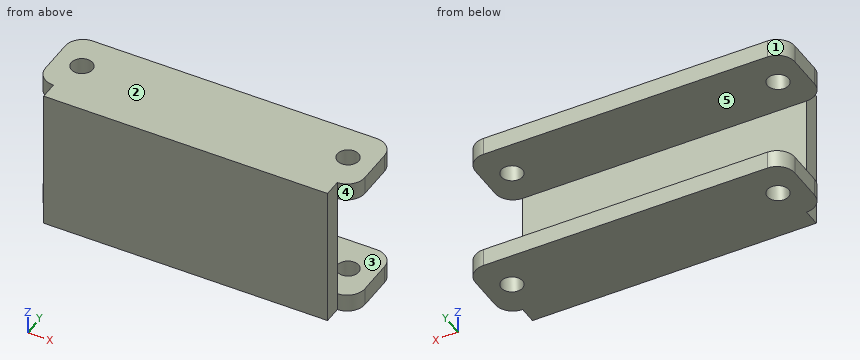
from build123d import *

# Parameters (mm, degrees)
SKETCH2_W           = 900
SKETCH2_H           = 200
BOSS_EXTRUDE1_DEPTH = 400
SKETCH3_W           = 1697.05478925
SKETCH3_H           = 300
CUT_EXTRUDE1_DEPTH  = 400
FILLET1_R           = 50
FILLET2_R           = 50
SKETCH4_R           = 30
CUT_EXTRUDE3_DEPTH  = 611.327780787
SKETCH4_2_W         = 800
SKETCH4_2_H         = 400
BOSS_EXTRUDE2_DEPTH = 50


with BuildPart() as part:
    # Sketch2 → Boss-Extrude1 (new body)
    with BuildSketch(Plane.XY):
        Rectangle(SKETCH2_W, SKETCH2_H)
    extrude(amount=BOSS_EXTRUDE1_DEPTH)

    # Sketch3 → Cut-Extrude1 (cut)
    with BuildSketch(Plane(origin=(0, 100, 0), x_dir=(1, 0, 0), z_dir=(0, 1, 0))):
        with Locations((0, -200)):
            Rectangle(SKETCH3_W, SKETCH3_H)
    extrude(amount=-CUT_EXTRUDE1_DEPTH, mode=Mode.SUBTRACT)


with BuildPart() as cut_extrude1_piece_1:
    # of the separate pieces the step leaves, piece 1, a body of its own (cut_extrude1_pieces)
    add(part.part.solids().sort_by_distance((-450, -100, 0))[0])

    # Fillet2
    fillet2_edges = [cut_extrude1_piece_1.edges().sort_by_distance(p)[0] for p in [
        (450, -100, 25),
        (-450, -100, 25),
        (-450, 100, 25),
        (450, 100, 25),
    ]]
    fillet(fillet2_edges, radius=FILLET2_R)


with BuildPart() as cut_extrude1_piece_2:
    # of the separate pieces the step leaves, piece 2, a body of its own (cut_extrude1_pieces)
    add(part.part.solids().sort_by_distance((-450, -100, 350))[0])

    # Fillet1
    fillet1_edges = [cut_extrude1_piece_2.edges().sort_by_distance(p)[0] for p in [
        (450, -100, 375),
        (450, 100, 375),
        (-450, 100, 375),
        (-450, -100, 375),
    ]]
    fillet(fillet1_edges, radius=FILLET1_R)


with BuildPart() as cut_extrude3_tool:
    # Sketch4 → Cut-Extrude3 (new, through all)
    with BuildSketch(Plane.XY.offset(400)):
        with Locations((-375, 0)):
            Circle(SKETCH4_R)
        with Locations((375, 0)):
            Circle(SKETCH4_R)
    extrude(amount=-CUT_EXTRUDE3_DEPTH)


with BuildPart() as cut_extrude1_piece_1_1:
    add(cut_extrude1_piece_1.part)

    # Cut-Extrude3: cut by cut_extrude3_tool
    add(cut_extrude3_tool.part, mode=Mode.SUBTRACT)



with BuildPart() as cut_extrude1_piece_2_1:
    add(cut_extrude1_piece_2.part)

    # Cut-Extrude3: cut by cut_extrude3_tool
    add(cut_extrude3_tool.part, mode=Mode.SUBTRACT)


with BuildPart() as cut_extrude1_piece_1_2:
    add(cut_extrude1_piece_1_1.part)

    add(cut_extrude1_piece_2_1.part)  # Boss-Extrude2 merges Cut-Extrude1 piece 2
    # Sketch4 2 → Boss-Extrude2 (add)
    with BuildSketch(Plane.XZ.offset(100)):
        with Locations((0, 200)):
            Rectangle(SKETCH4_2_W, SKETCH4_2_H)
    extrude(amount=BOSS_EXTRUDE2_DEPTH)


solid = cut_extrude1_piece_1_2.part
CAD build for the part. Positions are in the model's coordinates, mm. Face numbers are marked on the shaded views. A direction names the side the tool comes from. Give positions to 0.01 mm unless a question says otherwise; leave off trailing zeros. Order: outer loops, then holes, each group sorted by start corner. A loop starts at its lowest first (then second) coordinate and runs counter-clockwise, first axis right, second up. Notation, with made-up numbers: (-16, 26) - (35, 26) arc R23 ccw to (35, 51) - close; hole circle Ø10 at (6.25, -13.5). An arc over 180 degrees is marked (long way). Write each question's results on one line, items separated by ' | '.
1. Saw through at C-C on x = -189.5. List the corners of the cut face in (y, z).
Calculated:
outline: (-150, 0) - (100, 0) - (100, 50) - (-100, 50) - (-100, 350) - (100, 350) - (100, 400) - (-150, 400) - close
2. Saw through at D-D on z = 36. List the corners of the cut face in (x, y).
Calculated:
outline: (-450, -50) arc R50 ccw to (-400, -100) - (-400, -150) - (400, -150) - (400, -100) arc R50 ccw to (450, -50) - (450, 50) arc R50 ccw to (400, 100) - (-400, 100) arc R50 ccw to (-450, 50) - close; hole circle Ø60 at (-375, 0); hole circle Ø60 at (375, 0)
3. Pull direction Z, two halves, no side cores. Call the marked faces 1, 2 and 3: released by +Z, released by -Z, zero draft, split by the parting line, or undercut.
Calculated:
face 1: zero draft | face 2: released by +Z | face 3: undercut
4. Saw through at B-B on y = 0. List the corners of the cut face in (x, z), and give its area (3 significant figures).
Calculated:
outline: (-450, 0) - (-405, 0) - (-405, 50) - (-450, 50) - close; (-450, 350) - (-405, 350) - (-405, 400) - (-450, 400) - close; (-345, 0) - (345, 0) - (345, 50) - (-345, 50) - close; (-345, 350) - (345, 350) - (345, 400) - (-345, 400) - close; (405, 0) - (450, 0) - (450, 50) - (405, 50) - close; (405, 350) - (450, 350) - (450, 400) - (405, 400) - close | area: 78,000 mm2
5. 3-axis set-ups, long thin cutter, end or side, ignore diameter. For the marked faces 4 and 5: which of +Z, -Z, +X, -X, +Y, -Y reach the whole face in a straight line?
Calculated:
face 4: +Z, -Z, +X, -Y | face 5: +X, -X, +Y
6. Probe L1, parallel to Z at x = -249.5, y = -61; L2, parallel to Y at x = -375, z = 12; L3, parallel to X at y = 27, z = 358. List the from-to ranges inside material, lowest first. Write a range as from..to.
Calculated:
L1: z = 0..50, 350..400 | L2: y = -150..-30, 30..100 | L3: x = -450..-388.08, -361.92..361.92, 388.08..450
7. Saw through at A-A on x = 375. List the corners of the cut face in (y, z), and give its area (3 significant figures).
Calculated:
outline: (-150, 0) - (-30, 0) - (-30, 50) - (-100, 50) - (-100, 350) - (-30, 350) - (-30, 400) - (-150, 400) - close; (30, 0) - (100, 0) - (100, 50) - (30, 50) - close; (30, 350) - (100, 350) - (100, 400) - (30, 400) - close | area: 34,000 mm2
8. Pin check, flat tips, straight feed: pin 1 (6 mm diameter, centred on x = 105, z = 285.5, fed in from +Y); pin 2 (25 mm diameter, centred on y = -136.5, z = 111, fed in from +X). Stop position of each tip, or through.
Calculated:
pin 1: stops at y = -100 | pin 2: stops at x = 400
